```python
from build123d import *

# Parameters (mm, degrees)
F0_W     = 21
F0_H     = 18
F0_W_2   = 17
F0_H_2   = 14
F1_DEPTH = 2.5
F2_R     = 3
F3_DEPTH = 1
F4_W     = 5
F4_H     = 1
F5_DEPTH = 25
F6_R     = 2


with BuildPart() as f1:
    # F0 (on Top) → F1 (new body, symmetric)
    with BuildSketch(Plane.XY):
        Rectangle(F0_W, F0_H)
        Rectangle(F0_W_2, F0_H_2, mode=Mode.SUBTRACT)
        Rectangle(F0_W_2, F0_H_2)
    extrude(amount=F1_DEPTH, both=True)

    # F2
    f2_edges = [f1.edges().sort_by_distance(p)[0] for p in [
        (10.5, -9, 0),
        (10.5, 9, 0),
        (-10.5, 9, 0),
        (-10.5, -9, 0),
    ]]
    fillet(f2_edges, radius=F2_R)

    # F0 (on Top) → F3 (cut, symmetric)
    with BuildSketch(Plane.XY):
        Rectangle(F0_W, F0_H)
        Rectangle(F0_W_2, F0_H_2, mode=Mode.SUBTRACT)
    extrude(amount=F3_DEPTH, both=True, mode=Mode.SUBTRACT)

    # F4 (on face) → F5 (cut)
    with BuildSketch(Plane.XY.offset(2.5)):
        Polygon((-5.5, -0.5), (-5.5, -4), (5.5, -4), (5.5, 4), (-5.5, 4), (-5.5, 0.5), align=None)
        with Locations((-8, 0)):
            Rectangle(F4_W, F4_H)
    extrude(amount=-F5_DEPTH, mode=Mode.SUBTRACT)

    # F6
    f6_edges = [f1.edges().sort_by_distance(p)[0] for p in [
        (-5.5, -4, 0),
        (5.5, -4, 0),
        (5.5, 4, 0),
        (-5.5, 4, 0),
    ]]
    fillet(f6_edges, radius=F6_R)


solid = f1.part
```
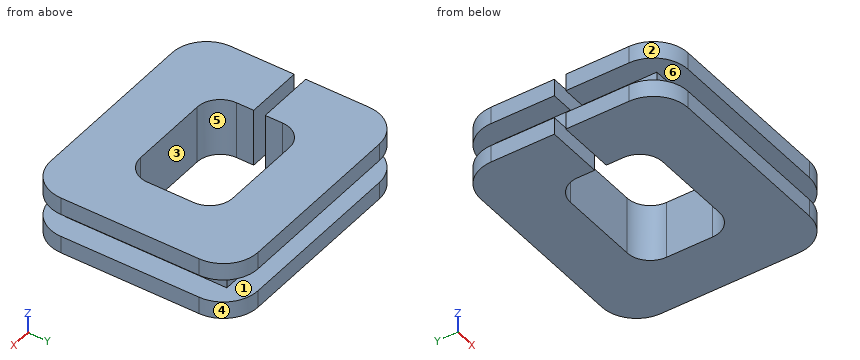
Part model, mm, in its own coordinate system. Face numbers are marked on the shaded views. A direction names the side the tool comes from. Round coordinates to 2 decimals unless told otherwise and drop trailing zeros. Write each loop counter-clockwise with the first axis right and the second up, starting at its lowest first coordinate (ties: lowest second). Pieces come first, ordered by that corner, then holes. Notation, with made-up numbers: (45, 46.5) -> (74, 46.5) arc R27 cw to (74, 71.5) -> close; hole circle Ø8 at (-11.75, -34). An arc over 180 degrees is marked (long way). Return JSON: item names as keys, results as strings. Group by question number.
Q1. Probe L1, parallel to X at y = -2, z = -1.9; L2, parallel to Y at x = 0, z = -1.45; L3, parallel to Z at x = -3, y = 8. List the from-to ranges inside material, lowest first. Write a range as [from, to].
Q2. Pin check, flat tips, straight feed: pin 1 (2.5 mm diameter, centred on x = -9, z = 0.5, fed in from -Y); pin 2 (1.6 mm diameter, centred on x = -2.5, z = 0, fed in from +Y); pin 3 (0.6 mm diameter, centred on y = 2.5, z = 0, fed in from -X). Stop position of each tip, or through.
Q3. Which spindle directions (+Z, -Z, +X, -X, +Y, -Y) get a long thin tool onto all of the face, cutting with end or side? Do the marked faces 1, 2 and 3. Say none if no direction does.
Q4. Saw through at D-D on x = 6. Write the cut outline in (y, z).
Q5. Saw through at A-A on x = -7.25. Write the cut outline in (y, z).
Q6. Mould opens along X. For the marked faces 4, 5 and 6 say: pulls with the +X half, pulls with the -X half, needs draft (parallel to the pull), parting line crosses it, or undercut.
Q7. Saw through at C-C on y = 0.25. Write the cut outline in (x, z).
Q8. Saw through at B-B on z = 1.65. Write the cut outline in (x, y), plus the area to 3 significant figures.
Answer:
{
 "1": {"L1": "[-10.5, -5.5], [5.5, 10.5]", "L2": "[-9, -4], [4, 9]", "L3": "[-2.5, -1], [1, 2.5]"},
 "2": {"pin 1": "y = -8.98", "pin 2": "y = 7", "pin 3": "x = -8.5"},
 "3": {"face 1": "none", "face 2": "+Z, -Z, -X, -Y", "face 3": "+Z, -Z"},
 "4": {"outline": "(-9, -2.5) -> (9, -2.5) -> (9, -1) -> (7, -1) -> (7, 1) -> (9, 1) -> (9, 2.5) -> (-9, 2.5) -> (-9, 1) -> (-7, 1) -> (-7, -1) -> (-9, -1) -> close"},
 "5": {"outline": "(-9, -2.5) -> (-0.5, -2.5) -> (-0.5, 2.5) -> (-9, 2.5) -> (-9, 1) -> (-7, 1) -> (-7, -1) -> (-9, -1) -> close; (0.5, -2.5) -> (9, -2.5) -> (9, -1) -> (7, -1) -> (7, 1) -> (9, 1) -> (9, 2.5) -> (0.5, 2.5) -> close"},
 "6": {"face 4": "pulls with the +X half", "face 5": "undercut", "face 6": "needs draft"},
 "7": {"outline": "(5.5, -2.5) -> (10.5, -2.5) -> (10.5, -1) -> (8.5, -1) -> (8.5, 1) -> (10.5, 1) -> (10.5, 2.5) -> (5.5, 2.5) -> close"},
 "8": {"outline": "(-10.5, -6) arc R3 ccw to (-7.5, -9) -> (7.5, -9) arc R3 ccw to (10.5, -6) -> (10.5, 6) arc R3 ccw to (7.5, 9) -> (-7.5, 9) arc R3 ccw to (-10.5, 6) -> (-10.5, 0.5) -> (-5.5, 0.5) -> (-5.5, 2) arc R2 cw to (-3.5, 4) -> (3.5, 4) arc R2 cw to (5.5, 2) -> (5.5, -2) arc R2 cw to (3.5, -4) -> (-3.5, -4) arc R2 cw to (-5.5, -2) -> (-5.5, -0.5) -> (-10.5, -0.5) -> close", "area": "281 mm2"}
}
